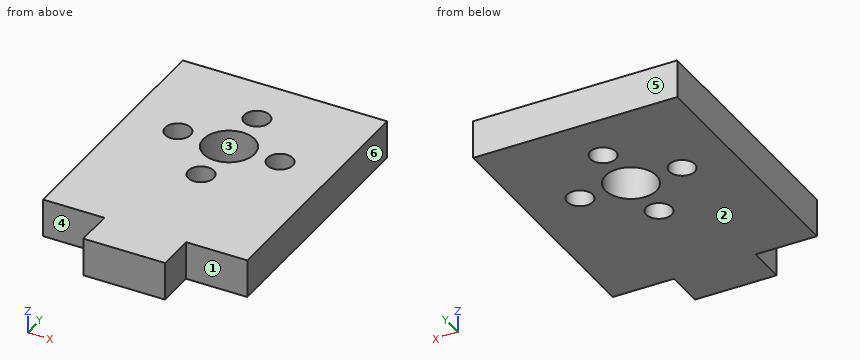
```python
from build123d import *

# Parameters (mm, degrees)
SKETCH1_R           = 3.175
SKETCH1_R_2         = 1.5875
BOSS_EXTRUDE1_DEPTH = 4.7625


with BuildPart() as part:
    # Sketch1 → Boss-Extrude1 (new body)
    with BuildSketch(Plane.XY):
        Polygon((25.4, 0), (25.4, 31.75), (0, 31.75), (0, 0), (7.62, 0), (7.62, -4.7625), (17.78, -4.7625), (17.78, 0), align=None)
        with Locations(Location((12.7, 19.05, 0), (0, 0, 180))):
            Circle(SKETCH1_R, mode=Mode.SUBTRACT)
        with Locations(Location((12.7, 25.4, 0), (0, 0, 180))):
            Circle(SKETCH1_R_2, mode=Mode.SUBTRACT)
        with Locations(Location((19.05, 19.05, 0), (0, 0, 180))):
            Circle(SKETCH1_R_2, mode=Mode.SUBTRACT)
        with Locations(Location((6.35, 19.05, 0), (0, 0, 180))):
            Circle(SKETCH1_R_2, mode=Mode.SUBTRACT)
        with Locations(Location((12.7, 12.7, 0), (0, 0, 180))):
            Circle(SKETCH1_R_2, mode=Mode.SUBTRACT)
    extrude(amount=BOSS_EXTRUDE1_DEPTH)


solid = part.part
```
Build history of the part. All positions in model axes, mm. Face numbers are marked on the shaded views. A direction names the side the tool comes from. Round coordinates to 2 decimals unless told otherwise and drop trailing zeros. Order: outer loops, then holes, each group sorted by start corner. A loop starts at its lowest first (then second) coordinate and runs counter-clockwise, first axis right, second up. Notation, with made-up numbers: (-13, 36.25) - (-7, 36.25) arc R25 cw to (-7, 68.25) - close; hole circle Ø1 at (-28.75, -36). An arc over 180 degrees is marked (long way). Use a Markdown table: item, result.
1) Wall check: L1, parallel to X at y = 19.05, z = 1.3 (1 decimal); L2, parallel to Y at x = 6.35, z = 1.7; L3, parallel to X at y = 12.7, z = 2.2. Give the ranges that are in metal, low to high.
Recorded:
| item | result |
|---|---|
| L1 | x = 0 to 4.8, 7.9 to 9.5, 15.9 to 17.5, 20.6 to 25.4 |
| L2 | y = 0 to 17.46, 20.64 to 31.75 |
| L3 | x = 0 to 11.11, 14.29 to 25.4 |
2) Pull direction Y, two halves, no side cores. Call the marked faces 3, 4, 5 and 6: pulls with the +Y half, pulls with the -Y half, needs draft (parallel to the pull), parting line crosses it, or undercut.
Recorded:
| item | result |
|---|---|
| face 3 | undercut |
| face 4 | pulls with the -Y half |
| face 5 | pulls with the +Y half |
| face 6 | needs draft |
3) Tool access for the marked faces 1 and 2: list every direction of +Z, -Z, +X, -X, +Y, -Y with a clear straight run to the whole face (end or side of a thin tool).
Recorded:
| item | result |
|---|---|
| face 1 | +Z, -Z, +X, -Y |
| face 2 | -Z, +X, -X, +Y, -Y |
4) Saw through at A-A on x = 19.05. Write the cut outline in (y, z), and give its area (3 significant figures).
Recorded:
| item | result |
|---|---|
| outline | (0, 0) - (17.46, 0) - (17.46, 4.76) - (0, 4.76) - close; (20.64, 0) - (31.75, 0) - (31.75, 4.76) - (20.64, 4.76) - close |
| area | 136 mm² |
5) Saw through at D-D on x = 7.25. Write the cut outline in (y, z), and give its area (3 significant figures).
Recorded:
| item | result |
|---|---|
| outline | (0, 0) - (17.74, 0) - (17.74, 4.76) - (0, 4.76) - close; (20.36, 0) - (31.75, 0) - (31.75, 4.76) - (20.36, 4.76) - close |
| area | 139 mm² |
6) Saw through at B-B on z = 1.55. Give the number of separate pieces and of enclosed holes in the cut face, and give its area (4 significant figures).
Recorded:
| item | result |
|---|---|
| separate pieces | 1 |
| enclosed holes | 5 |
| area | 791.5 mm² |
7) Saw through at C-C on y = 19.05. Write the cut outline in (x, z) (1 decimal), and give its area (3 significant figures).
Recorded:
| item | result |
|---|---|
| outline | (0, 0) - (4.8, 0) - (4.8, 4.8) - (0, 4.8) - close; (7.9, 0) - (9.5, 0) - (9.5, 4.8) - (7.9, 4.8) - close; (15.9, 0) - (17.5, 0) - (17.5, 4.8) - (15.9, 4.8) - close; (20.6, 0) - (25.4, 0) - (25.4, 4.8) - (20.6, 4.8) - close |
| area | 60.5 mm² |
8) Flat gauge pins, fed straight in: pin 1 Ø1.5 at (y, z) = (12, 3.5) entering from -X; pin 2 Ø2 at (x, z) = (3, 1) entering from -Y; pin 3 Ø1.9 at (x, y) = (12.7, 25.4) entering from +Z; pin 4 Ø2.5 at (y, z) = (-2.5, 1.5) entering from +X. Where does each tip first touch, or does it go through?
Recorded:
| item | result |
|---|---|
| pin 1 | stops at x = 0 |
| pin 2 | stops at y = 0 |
| pin 3 | passes through |
| pin 4 | stops at x = 17.78 |
